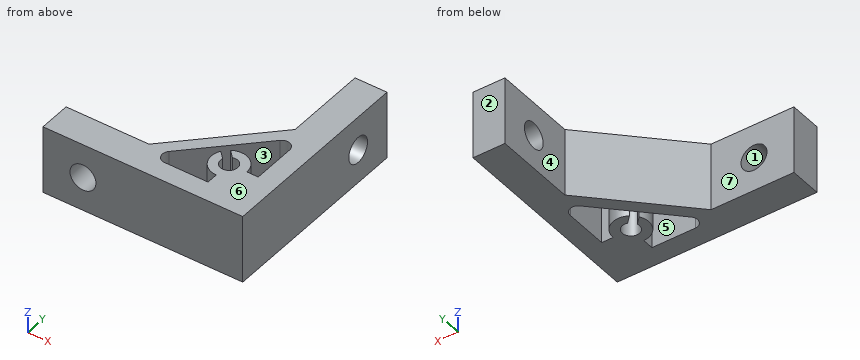
```python
from build123d import *

# Parameters (mm, degrees)
EXTRUDE_1_DEPTH     = 8.5
SKETCH_3_R          = 3.25
CUT_EXTRUDE_1_DEPTH = 17


with BuildPart() as part:
    # 草图1 → 凸台-拉伸1 (new, symmetric)
    with BuildSketch(Plane.XY):
        Polygon((0, 0), (50, 0), (50, 50), (42, 50), (42, 29.242640687), (20.757359313, 8), (0, 8), align=None)
        with BuildLine():
            Line((37.061279898, 14.352933665), (35.340960992, 16.07325257))
            ThreePointArc((35.340960992, 16.07325257), (39.856939547, 16.192314452), (42.15, 12.3))
            Line((42.15, 12.3), (45, 12.3))
            Line((45, 12.3), (45, 23.171572875))
            ThreePointArc((45, 23.171572875), (43.765366865, 25.01933194), (41.585786438, 24.585786438))
            Line((41.585786438, 24.585786438), (25.414213562, 8.414213562))
            ThreePointArc((25.414213562, 8.414213562), (24.98066806, 6.234633135), (26.828427125, 5))
            Line((26.828427125, 5), (37.7, 5))
            Line((37.7, 5), (37.7, 7.85))
            ThreePointArc((37.7, 7.85), (33.807685548, 10.143060453), (33.92674743, 14.659039008))
            Line((33.92674743, 14.659039008), (35.647066335, 12.938720102))
            ThreePointArc((35.647066335, 12.938720102), (39.22027958, 10.77972042), (37.061279898, 14.352933665))
        make_face(mode=Mode.SUBTRACT)
    extrude(amount=EXTRUDE_1_DEPTH, both=True)

    # 草图3 → 切除-拉伸1 (cut)
    with BuildSketch(Plane(origin=(0, 8, 0), x_dir=(1, 0, 0), z_dir=(0, 1, 0))):
        with Locations(Location((10, 0, 0), (0, 0, 270))):
            Circle(SKETCH_3_R)
    cut_extrude_1 = extrude(amount=-CUT_EXTRUDE_1_DEPTH, mode=Mode.SUBTRACT)

    # 镜向1: 切除-拉伸1 across plane
    add(cut_extrude_1.mirror(Plane(origin=(25, 25, 0), x_dir=(0, 0, 1), z_dir=(-0.7071067811865486, -0.7071067811865465, 0))), mode=Mode.SUBTRACT)


solid = part.part
```
Input: part model. Units: mm. Frame: model coordinates. Face numbers are marked on the shaded views. A direction names the side the tool comes from. Coordinates: 2 decimals unless noted, no trailing zeros. Write each loop counter-clockwise with the first axis right and the second up, starting at its lowest first coordinate (ties: lowest second). Pieces come first, ordered by that corner, then holes. Notation, with made-up numbers: (28.5, 68.5) - (86.5, 68.5) arc R34 ccw to (86.5, 103.5) - close; hole circle Ø5 at (22, -16.5). An arc over 180 degrees is marked (long way). Put each result on its own line as item: value. Start each with the question number.
1) Mould query, pull axis X, two halves, no side actions, for the marked faces 1, 2, 3 and 4. Classes: pulls with the +X half, pulls with the -X half, needs draft (parallel to the pull), parting line crosses it, or undercut.
2) Cut plane D-D (y = 24). Return the cut outline in (x, z).
3) Cut plane C-C (z = -6). Return the cut outline in (x, y).
4) Cut plane A-A (z = 0). Return the cut outline in (x, y), plus the area to 3 significant figures.
5) Ray query, L1, parallel to Y at x = 48, z = 0; L2, parallel to X at y = 6.75, z = 0; L3, parallel to Y at x = 39.5, z = 0.25. Return the intervals inside material, ascending.
6) Contact query for flat-ended pins moving along their axis: pin 1 (2 mm diameter, centred on x = 19, z = 5.5, fed in from +Y); pin 2 (7.5 mm diameter, centred on y = 40, z = 0, fed in from -X); pin 3 (1.5 mm diameter, centred on x = 33, z = -3.5, fed in from -Y); pin 4 (8.5 mm diameter, centred on x = 33.5, z = -1.5, fed in from +Y). Output: stop coordinate, or through.
7) Cut plane B-B (y = 40). Return the cut outline in (x, z).
8) Reachability of the marked faces 5, 6 and 7 from +Z, -Z, +X, -X, +Y, -Y: full face, straight path, thin tool, end or side. Return the list, or none.
Resolved:
1. face 1: undercut
1. face 2: needs draft
1. face 3: undercut
1. face 4: pulls with the -X half
2. outline: (36.76, -8.5) - (41, -8.5) - (41, 8.5) - (36.76, 8.5) - close; (44.82, -8.5) - (50, -8.5) - (50, 8.5) - (44.82, 8.5) - close
3. outline: (0, 0) - (50, 0) - (50, 50) - (42, 50) - (42, 29.24) - (20.76, 8) - (0, 8) - close; hole (25.41, 8.41) arc R2 ccw to (26.83, 5) - (37.7, 5) - (37.7, 7.85) arc R4.45 cw to (33.93, 14.66) - (35.65, 12.94) arc R2.15 ccw (long way) to (37.06, 14.35) - (35.34, 16.07) arc R4.45 cw to (42.15, 12.3) - (45, 12.3) - (45, 23.17) arc R2 ccw to (41.59, 24.59) - close
4. outline: (0, 0) - (6.75, 0) - (6.75, 8) - (0, 8) - close; (13.25, 0) - (50, 0) - (50, 36.75) - (42, 36.75) - (42, 29.24) - (20.76, 8) - (13.25, 8) - close; (42, 43.25) - (50, 43.25) - (50, 50) - (42, 50) - close; hole (25.41, 8.41) arc R2 ccw to (26.83, 5) - (37.7, 5) - (37.7, 7.85) arc R4.45 cw to (33.93, 14.66) - (35.65, 12.94) arc R2.15 ccw (long way) to (37.06, 14.35) - (35.34, 16.07) arc R4.45 cw to (42.15, 12.3) - (45, 12.3) - (45, 23.17) arc R2 ccw to (41.59, 24.59) - close
4. area: 684 mm2
5. L1: y = 0 to 36.75, 43.25 to 50
5. L2: x = 0 to 6.75, 13.25 to 24.84, 37.7 to 50
5. L3: y = 0 to 11.12, 13.48 to 16.37, 22.5 to 26.74
6. pin 1: stops at y = 8
6. pin 2: stops at x = 42
6. pin 3: stops at y = 0
6. pin 4: stops at y = 24.99
7. outline: (42, -8.5) - (50, -8.5) - (50, -3.25) - (42, -3.25) - close; (42, 3.25) - (50, 3.25) - (50, 8.5) - (42, 8.5) - close
8. face 5: +Z, -Z
8. face 6: +Z, +X, -X, +Y, -Y
8. face 7: +Z, -Z, -X, +Y
